Design review of the part built by this model. Coordinates are the model's own, in mm. A direction names the side the tool comes from. Give positions to 0.01 mm unless a question says otherwise; leave off trailing zeros. Loops run counter-clockwise (first coordinate to the right, second up) from the corner with the lowest first, then second, coordinate; pieces in that order, holes last.
from build123d import *

# Parameters (mm, degrees)
SKETCH3_R           = 1.25
BOSS_EXTRUDE1_DEPTH = 3
SKETCH4_W           = 45
SKETCH4_H           = 3
BOSS_EXTRUDE2_DEPTH = 10
FILLET1_R           = 2
FILLET2_R           = 2
SKETCH5_R           = 1.5
CUT_EXTRUDE1_DEPTH  = 29.702134145


with BuildPart() as part:
    # Sketch3 → Boss-Extrude1 (new body)
    with BuildSketch(Plane.XY):
        with BuildLine():
            Line((-12.2, 6.25), (-12.2, -5))
            ThreePointArc((-12.2, -5), (-12.492893219, -5.707106781), (-13.2, -6))
            Line((-13.2, -6), (-15.6, -6))
            ThreePointArc((-15.6, -6), (-16.208761429, -5.79335334), (-16.565925826, -5.258819045))
            Line((-16.565925826, -5.258819045), (-19.386481515, 5.26763809))
            ThreePointArc((-19.386481515, 5.26763809), (-20.100810309, 6.336706681), (-21.318333167, 6.75))
            Line((-21.318333167, 6.75), (-21.5, 6.75))
            ThreePointArc((-21.5, 6.75), (-22.207106781, 7.042893219), (-22.5, 7.75))
            Line((-22.5, 7.75), (-22.5, 11.75))
            Line((-22.5, 11.75), (22.5, 11.75))
            Line((22.5, 11.75), (22.5, 7.75))
            ThreePointArc((22.5, 7.75), (22.207106781, 7.042893219), (21.5, 6.75))
            Line((21.5, 6.75), (21.318333167, 6.75))
            ThreePointArc((21.318333167, 6.75), (20.100810309, 6.336706681), (19.386481515, 5.26763809))
            Line((19.386481515, 5.26763809), (16.565925826, -5.258819045))
            ThreePointArc((16.565925826, -5.258819045), (16.208761429, -5.79335334), (15.6, -6))
            Line((15.6, -6), (13.2, -6))
            ThreePointArc((13.2, -6), (12.492893219, -5.707106781), (12.2, -5))
            Line((12.2, -5), (12.2, 6.25))
            ThreePointArc((12.2, 6.25), (12.053553391, 6.603553391), (11.7, 6.75))
            Line((11.7, 6.75), (-11.7, 6.75))
            ThreePointArc((-11.7, 6.75), (-12.053553391, 6.603553391), (-12.2, 6.25))
        make_face()
        with Locations((-14.4, 0)):
            Circle(SKETCH3_R, mode=Mode.SUBTRACT)
        with Locations((14.4, 0)):
            Circle(SKETCH3_R, mode=Mode.SUBTRACT)
    extrude(amount=BOSS_EXTRUDE1_DEPTH)

    # Sketch4 → Boss-Extrude2 (add)
    with BuildSketch(Plane(origin=(0, 0, 0), x_dir=(-1, 0, 0), z_dir=(0, 0, -1))):
        with Locations((0, 10.25)):
            Rectangle(SKETCH4_W, SKETCH4_H)
    extrude(amount=BOSS_EXTRUDE2_DEPTH)

    # Fillet1
    fillet1_edges = [part.edges().sort_by_distance(p)[0] for p in [
        (0, 8.75, 0),
    ]]
    fillet(fillet1_edges, radius=FILLET1_R - 0.0001)  # a hair under: the kernel refuses the full size

    # Fillet2
    fillet2_edges = [part.edges().sort_by_distance(p)[0] for p in [
        (22.5, 10.25, -10),
        (-22.5, 10.25, -10),
    ]]
    fillet(fillet2_edges, radius=FILLET2_R)

    # Sketch5 → Cut-Extrude1 (cut, through all)
    with BuildSketch(Plane.XZ.offset(-8.75)):
        with Locations(Location((-18.5, -6, 0), (0, 0, 270))):
            Circle(SKETCH5_R)
    cut_extrude1 = extrude(amount=-CUT_EXTRUDE1_DEPTH, mode=Mode.SUBTRACT)

    # Mirror1: Cut-Extrude1 across plane
    add(cut_extrude1.mirror(Plane(origin=(0, 0, 0), x_dir=(0, 0, 1), z_dir=(1, 0, 0))), mode=Mode.SUBTRACT)


solid = part.part
Q1. Take a section at D-D (y = 0). Give the boundary of the cut face in (x, z), plus the area to 3 significant figures.
Results:
outline: (-17.98, 0) - (-15.65, 0) - (-15.65, 3) - (-17.98, 3) - close; (-13.15, 0) - (-12.2, 0) - (-12.2, 3) - (-13.15, 3) - close; (12.2, 0) - (13.15, 0) - (13.15, 3) - (12.2, 3) - close; (15.65, 0) - (17.98, 0) - (17.98, 3) - (15.65, 3) - close
area: 19.7 mm2
Q2. Take a section at C-C (y = 2.25). Give the boundary of the cut face in (x, z), plus the area to 3 significant figures.
Results:
outline: (-18.58, 0) - (-12.2, 0) - (-12.2, 3) - (-18.58, 3) - close; (12.2, 0) - (18.58, 0) - (18.58, 3) - (12.2, 3) - close
area: 38.3 mm2
Q3. Tool access review of faces 1 (the face through (12.501, -5.715, 1.479)), 2 (the face through (0, 11.75, -3)), 3 (the face through (0, 8.75, -6)): name each direction out of +Z, -Z, +X, -X, +Y, -Y from which nothing blocks a thin tool from reaching the whole face with its end or side.
Results:
face 1: +Z, -Z, -Y
face 2: +Z, -Z, +X, -X, +Y
face 3: -Z, +X, -X, -Y
Q4. Take a section at B-B (z = -6). Give the boundary of the cut face in (x, y).
Results:
outline: (-22.5, 8.75) - (-20, 8.75) - (-20, 11.75) - (-22.5, 11.75) - close; (-17, 8.75) - (17, 8.75) - (17, 11.75) - (-17, 11.75) - close; (20, 8.75) - (22.5, 8.75) - (22.5, 11.75) - (20, 11.75) - close
Q5. Insertion check: pin 1 (5 mm diameter, centred on x = -6, z = -8.5, fed in from -Y); pin 2 (10 mm diameter, centred on x = -11.5, y = 2, fed in from -Z); pin 3 (0.9 mm diameter, centred on y = -0.5, z = 1, fed in from +X). Each pin has a flat end and moves straight along its axis. Give the tip position at first contact, or say it passes through.
Results:
pin 1: stops at y = 8.75
pin 2: stops at z = -0.02
pin 3: stops at x = 17.96
Q6. Wall thickness on line 1 (X direction, y = 9.8, z = -6); line 2 (Z direction, x = 18.5, y = 10.15); line 3 (Y direction, x = 14.4, z = 1.85): over which ranges is each line inside the solid? List them lowest first.
Results:
line 1: x = -22.5 to -20, -17 to 17, 20 to 22.5
line 2: z = -10 to -7.5, -4.5 to 3
line 3: y = -6 to -1.25, 1.25 to 11.75
Q7. Take a section at A-A (x = 14.4). Give the boundary of the cut face in (y, z).
Results:
outline: (-6, 0) - (-1.25, 0) - (-1.25, 3) - (-6, 3) - close; (1.25, 0) - (6.75, 0) arc R2 cw to (8.75, -2) - (8.75, -10) - (11.75, -10) - (11.75, 3) - (1.25, 3) - close
Q8. Draft analysis for pull direction Y (two halves, no side actions). For faces 4 (the face through (-12.485, -5.699, 1.479)), 5 (the face through (15.59, 0.38, 1.48)), 6 (the face through (-15.65, 0.05, 1.48)), 7 (the face through (-12.2, 1, 1)), state which applies: pulls with the +Y half, pulls with the -Y half, needs draft (parallel to the pull), parting line crosses it, or undercut.
Results:
face 4: pulls with the -Y half
face 5: undercut
face 6: undercut
face 7: needs draft
